Here's how the part is built. I have some questions about the finished solid (model axes, mm). A direction names the side the tool comes from. Coordinates: 2 decimals unless noted, no trailing zeros. Write each loop counter-clockwise with the first axis right and the second up, starting at its lowest first coordinate (ties: lowest second). Pieces come first, ordered by that corner, then holes.
Item 1: I'm going to push flat-ended pins straight in: P1, Ø5.5, axis at x = 187, y = -41, coming from the +Z side; P2, Ø1, axis at x = 78, y = -8, coming from the +Z side; P3, Ø5, axis at x = 228.5, y = -44.5, coming from the -Z side. Where does each tip first touch, or does it pass through?
Item 2: I want a section at B-B (z = -28.5). Please give me the cut outline in (x, y), and give its area (3 significant figures).
Item 3: Please list where these lines run through material, in increasing order: line 1 (Z direction, x = 172.5, y = -15); line 2 (Z direction, x = -13, y = -4.5); line 3 (Z direction, x = 187, y = -38.5).
Item 4: I want a section at A-A (z = 30). Please give me the cut outline in (x, y), and give its area (3 significant figures).
Item 5: If we mould it in two halves opening along Z, with no side actions, what happens to faces 1 (the face through (226, -40.859, 0)), 2 (the face through (-25, -42, 2.5)), 3 (the face through (-27.667, -28, 0)), 4 (the face through (-20, -28, -7.5))? For each: pulls with the +Z half, pulls with the -Z half, needs draft (parallel to the pull), parting line crosses it, or undercut.
Item 6: For faces 5 (the face through (-22.667, -42, -5)), 6 (the face through (186, -42, -2.5)), 7 (the face through (-15, -36.859, 5)), 8 (the face through (-20, -46.859, 0)), which set-ups out of +Z, -Z, +X, -X, +Y, -Y let a thin tool reach every point of the face, with its end or its side?
from build123d import *

# Parameters (mm, degrees)
SWEEP2_PROFILE_R         = 39
CUT_EXTRUDE5_DEPTH       = 400
BOSS_EXTRUDE2_REACH      = 250.512
BOSS_EXTRUDE2_END_RADIUS = 39
SKETCH30_W               = 15
SKETCH30_H               = 15
SKETCH31_W               = 5
SKETCH31_H               = 5
CUT_EXTRUDE6_DEPTH       = 10
BOSS_EXTRUDE3_REACH      = 250.512
BOSS_EXTRUDE3_END_RADIUS = 39
CUT_EXTRUDE7_DEPTH       = 6


with BuildPart() as part:
    # Sweep2: sweep along a path in Sketch17
    with BuildLine(Plane.XY) as sweep2_path:
        Line((-56.942235333, 25.5), (234.524098388, 0))
    # Sweep2 profile (on start of the path) → Sweep2 (sweep)
    with BuildSketch(Plane(origin=(-56.942235333, 25.5, 0), x_dir=(0.08715574274765121, 0.9961946980917462, 0), z_dir=(0.9961946980917462, -0.08715574274765121, 0))):
        Circle(SWEEP2_PROFILE_R)
    sweep(path=sweep2_path.line)

    # Sketch25 → Cut-Extrude5 (cut)
    with BuildSketch(Plane(origin=(232.742624374, -20.362341152, 0), x_dir=(0, 0, -1), z_dir=(0.9961946980917462, -0.08715574274765125, 0))):
        with BuildLine():
            Line((40.377384308, 20.440121987), (40.377384308, 67.184416815))
            Line((40.377384308, 67.184416815), (-52.333834244, 67.184416815))
            Line((-52.333834244, 67.184416815), (-52.333834244, 20.440121987))
            Line((-52.333834244, 20.440121987), (-35, 20.440121987))
            ThreePointArc((-35, 20.440121987), (0, -14.559878013), (35, 20.440121987))
            Line((35, 20.440121987), (40.377384308, 20.440121987))
        make_face()
    extrude(amount=-CUT_EXTRUDE5_DEPTH, mode=Mode.SUBTRACT)

    # Boss-Extrude2: up to this cylinder (the profile starts outside it)
    boss_extrude2_end = Plane(origin=(90.766179518, 12.577188193, 0), z_dir=(0.9961946980917462, -0.08715574274765124, 0)) * Cylinder(BOSS_EXTRUDE2_END_RADIUS, 790.685640756, mode=Mode.PRIVATE)
    # Sketch30 → Boss-Extrude2 (add, up to the surface)
    with BuildSketch(Plane(origin=(0, -46.859203829, 0), x_dir=(1, 0, 0), z_dir=(0, 1, 0)), mode=Mode.PRIVATE) as boss_extrude2_sk1:
        with Locations((-20.166997814, 0)):
            Rectangle(SKETCH30_W, SKETCH30_H)
    boss_extrude2_tool1 = extrude(boss_extrude2_sk1.sketch, amount=BOSS_EXTRUDE2_REACH, mode=Mode.PRIVATE) - boss_extrude2_end
    add(boss_extrude2_tool1.solids().sort_by_distance((-20.166998, -46.859204, 0))[0])
    # Sketch30 → Boss-Extrude2 (add, up to the surface)
    with BuildSketch(Plane(origin=(0, -46.859203829, 0), x_dir=(1, 0, 0), z_dir=(0, 1, 0)), mode=Mode.PRIVATE) as boss_extrude2_sk2:
        with Locations((191.299335906, 0)):
            Rectangle(SKETCH30_W, SKETCH30_H)
    boss_extrude2_tool2 = extrude(boss_extrude2_sk2.sketch, amount=BOSS_EXTRUDE2_REACH, mode=Mode.PRIVATE) - boss_extrude2_end
    add(boss_extrude2_tool2.solids().sort_by_distance((191.299336, -46.859204, 0))[0])

    # Sketch31 → Cut-Extrude6 (cut)
    with BuildSketch(Plane.XZ.offset(46.859203829)):
        with Locations((-25.166997814, 5)):
            Rectangle(SKETCH31_W, SKETCH31_H)
        with Locations((-15.166997814, 5)):
            Rectangle(SKETCH31_W, SKETCH31_H)
        with Locations((-15.166997814, -5)):
            Rectangle(SKETCH31_W, SKETCH31_H)
        with Locations((-25.166997814, -5)):
            Rectangle(SKETCH31_W, SKETCH31_H)
        with Locations((186.299335906, -5)):
            Rectangle(SKETCH31_W, SKETCH31_H)
        with Locations((196.299335906, -5)):
            Rectangle(SKETCH31_W, SKETCH31_H)
        with Locations((196.299335906, 5)):
            Rectangle(SKETCH31_W, SKETCH31_H)
        with Locations((186.299335906, 5)):
            Rectangle(SKETCH31_W, SKETCH31_H)
    extrude(amount=-CUT_EXTRUDE6_DEPTH, mode=Mode.SUBTRACT)

    # Boss-Extrude3: up to this cylinder (the profile starts outside it)
    boss_extrude3_end = Plane(origin=(230.603306914, 0.343024806, 0), z_dir=(0.9961946980917462, -0.08715574274765124, 0)) * Cylinder(BOSS_EXTRUDE3_END_RADIUS, 580.024, mode=Mode.PRIVATE)
    # Sketch38 → Boss-Extrude3 (add, up to the surface)
    with BuildSketch(Plane(origin=(0, -46.859203829, 0), x_dir=(1, 0, 0), z_dir=(0, 1, 0)), mode=Mode.PRIVATE) as boss_extrude3_sk1:
        Polygon((231.473647391, 0), (231.473647391, -7.5), (221.473647391, -7.5), (221.473647391, 7.5), (231.473647391, 7.5), align=None)
    boss_extrude3_tool1 = extrude(boss_extrude3_sk1.sketch, amount=BOSS_EXTRUDE3_REACH, mode=Mode.PRIVATE) - boss_extrude3_end
    add(boss_extrude3_tool1.solids().sort_by_distance((226.473647, -46.859204, 0))[0])

    # Sketch39 → Cut-Extrude7 (cut)
    with BuildSketch(Plane.XZ.offset(46.859203829)):
        Polygon((231.473647391, 0), (231.473647391, 2.6), (221.473647391, 2.6), (221.473647391, -2.6), (231.473647391, -2.6), align=None)
    extrude(amount=-CUT_EXTRUDE7_DEPTH, mode=Mode.SUBTRACT)


solid = part.part
Answer:
1. P1: stops at z = 7.5
1. P2: stops at z = 32.79
1. P3: stops at z = -7.5
2. outline: (-59.26, -1.02) - (232.2, -26.52) - (232.75, -20.24) - (-58.71, 5.26) - close
2. area: 1,850 mm2
3. line 1: z = -33.27 to -28.48, 28.48 to 33.27
3. line 2: z = -29.02 to -23.37, 23.37 to 29.02
3. line 3: z = -2.5 to 2.5
4. outline: (-59.11, 0.67) - (232.35, -24.83) - (232.95, -17.96) - (-58.51, 7.54) - close
4. area: 2,020 mm2
5. face 1: undercut
5. face 2: pulls with the +Z half
5. face 3: needs draft
5. face 4: pulls with the -Z half
6. face 5: -Z, -X, -Y
6. face 6: -Z, -Y
6. face 7: +Z, -Y
6. face 8: +Z, -Z, +X, -X, -Y
